Verification items for the finished model (mm, model axes). A direction names the side the tool comes from. Round coordinates to 2 decimals unless told otherwise and drop trailing zeros. Order: outer loops, then holes, each group sorted by start corner. A loop starts at its lowest first (then second) coordinate and runs counter-clockwise, first axis right, second up.
```python
from build123d import *

# Parameters (mm, degrees)
F0_R     = 85
F1_DEPTH = 20
F2_R     = 53.5
F2_R_2   = 40
F3_DEPTH = 8
F4_R     = 5
F5_DEPTH = 20.001


with BuildPart() as f1:
    # F0 (on Top) → F1 (new body)
    with BuildSketch(Plane.XY):
        Circle(F0_R)
    extrude(amount=F1_DEPTH)

    # F2 (on face) → F3 (cut)
    with BuildSketch(Plane.XY.offset(20)):
        Circle(F2_R)
        Circle(F2_R_2, mode=Mode.SUBTRACT)
    extrude(amount=-F3_DEPTH, mode=Mode.SUBTRACT)

    # F4 (on face) → F5 (cut, through all)
    with BuildSketch(Plane.XY.offset(20)):
        Circle(F4_R)
    extrude(amount=-F5_DEPTH, mode=Mode.SUBTRACT)


solid = f1.part
```
1) Tool access check on faces 1 (the flat face through (20, -35, 12)), 2 (the flat face through (8, 1, 20)). Record the directions out of +Z, -Z, +X, -X, +Y, -Y that give a thin tool (end or side, any length) a straight path to the whole face; none if there is none.
2) Sectioned sample at D-D on y = -19.5. Record the cut outline in (x, z).
3) Go/stop test with flat-tipped pins: pin 1 Ø1 at (x, z) = (45.5, 3.5) entering from -Y; pin 2 Ø10 at (x, z) = (-7.5, 10.5) entering from -Y; pin 3 Ø4 at (x, z) = (-35.5, 17) entering from +Y. Record where each tip stops, or that it passes through.
4) Draft check along Y on faces 3 (the flat face through (-1, -55, 20)), 4 (the cylindrical face through (-67.453, -51.721, 9.86)), 5 (the cylindrical face through (-1.08, -4.88, 10.14)). Enter one of: released by +Y, released by -Y, zero draft, split by the parting line, or undercut.
5) Scan lines: probe 1 along Y at (x, z) = (0, 14); probe 2 along Y at (x, z) = (0, 7.5); probe 3 along Z at (x, y) = (-42, 14.5). Record each from-to range of solid material in increasing order.
6) Sectioned sample at A-A on y = 0. Record the cut outline in (x, z).
7) Sectioned sample at C-C on z = 9. Record the cut outline in (x, y).
Returned:
1. face 1: +Z
1. face 2: +Z, +X, -X, +Y, -Y
2. outline: (-82.73, 0) - (82.73, 0) - (82.73, 20) - (49.82, 20) - (49.82, 12) - (34.92, 12) - (34.92, 20) - (-34.92, 20) - (-34.92, 12) - (-49.82, 12) - (-49.82, 20) - (-82.73, 20) - close
3. pin 1: stops at y = -72.11
3. pin 2: stops at y = -84.96
3. pin 3: stops at y = 78.12
4. face 3: zero draft
4. face 4: split by the parting line
4. face 5: undercut
5. probe 1: y = -85 to -53.5, -40 to -5, 5 to 40, 53.5 to 85
5. probe 2: y = -85 to -5, 5 to 85
5. probe 3: z = 0 to 12
6. outline: (-85, 0) - (-5, 0) - (-5, 20) - (-40, 20) - (-40, 12) - (-53.5, 12) - (-53.5, 20) - (-85, 20) - close; (5, 0) - (85, 0) - (85, 20) - (53.5, 20) - (53.5, 12) - (40, 12) - (40, 20) - (5, 20) - close
7. outline: circle Ø170 at (0, 0); hole circle Ø10 at (0, 0)
